Geometry check sheet. Reference: the model listing, model coordinates, mm. A direction names the side the tool comes from. Coordinates: 2 decimals unless noted, no trailing zeros. Write each loop counter-clockwise with the first axis right and the second up, starting at its lowest first coordinate (ties: lowest second). Pieces come first, ordered by that corner, then holes.
from build123d import *

# Parameters (mm, degrees)
BOSS_EXTRUDE1_DEPTH             = 15
SKETCH4_R                       = 10.5
CUT_EXTRUDE2_DEPTH              = 2
M3_CLEARANCE_HOLE2_D            = 3.4
M3X0_5_TAPPED_HOLE1_D           = 2.5
M3X0_5_TAPPED_HOLE1_CSINK_D     = 10
M3X0_5_TAPPED_HOLE1_CSINK_ANGLE = 90


with BuildPart() as part:
    # Sketch1 → Boss-Extrude1 (new body)
    with BuildSketch(Plane.XY):
        with BuildLine():
            Line((0.6875, 12.48107943), (100.385, 6.989404481))
            ThreePointArc((100.385, 6.989404481), (107, 0), (100.385, -6.989404481))
            Line((100.385, -6.989404481), (0.6875, -12.48107943))
            ThreePointArc((0.6875, -12.48107943), (-12.5, 0), (0.6875, 12.48107943))
        make_face()
    extrude(amount=BOSS_EXTRUDE1_DEPTH)

    # Sketch4 → Cut-Extrude2 (cut)
    with BuildSketch(Plane.XY.offset(15)):
        Circle(SKETCH4_R)
    extrude(amount=-CUT_EXTRUDE2_DEPTH, mode=Mode.SUBTRACT)

    # M3 Clearance Hole2 (through all)
    with Locations(Plane.XY.offset(15)):
        with Locations((100, 0)):
            Hole(M3_CLEARANCE_HOLE2_D / 2)

    # M3x0.5 Tapped Hole1 (through all)
    with Locations(Plane(origin=(0, 0, 0), x_dir=(-1, 0, 0), z_dir=(0, 0, -1))):
        with Locations((0, 0)):
            CounterSinkHole(M3X0_5_TAPPED_HOLE1_D / 2, M3X0_5_TAPPED_HOLE1_CSINK_D / 2, counter_sink_angle=M3X0_5_TAPPED_HOLE1_CSINK_ANGLE)


solid = part.part
1. Sectioned sample at A-A, the plane y = 0. Record the boundary of the cut face in (x, z).
Computed values:
outline: (-12.5, 0) - (-5, 0) - (-1.25, 3.75) - (-1.25, 13) - (-10.5, 13) - (-10.5, 15) - (-12.5, 15) - close; (1.25, 3.75) - (5, 0) - (98.3, 0) - (98.3, 15) - (10.5, 15) - (10.5, 13) - (1.25, 13) - close; (101.7, 0) - (107, 0) - (107, 15) - (101.7, 15) - close
2. Access from +Z, -Z, +X, -X, +Y, -Y to the whole of each face (thin tool, end or side, straight path). Record for faces 1 (the cylindrical face through (10, 3.2, 14)), 2 (the conical face through (-0.31, -1.398, 3.568)).
Computed values:
face 1: +Z
face 2: -Z
3. Sectioned sample at C-C, the plane y = -9.25. Record the boundary of the cut face in (x, z).
Computed values:
outline: (-8.41, 0) - (59.35, 0) - (59.35, 15) - (4.97, 15) - (4.97, 13) - (-4.97, 13) - (-4.97, 15) - (-8.41, 15) - close
4. Sectioned sample at D-D, the plane x = 22. Record the boundary of the cut face in (y, z).
Computed values:
outline: (-11.31, 0) - (11.31, 0) - (11.31, 15) - (-11.31, 15) - close
5. Sectioned sample at B-B, the plane z = 7. Give the number of separate pieces and of enclosed holes in the cut face, and give its area (3 significant figures).
Computed values:
separate pieces: 1
enclosed holes: 2
area: 2,260 mm2
6. Gauge pin test, flat ends, axial feed: pin 1 Ø3 at (x, y) = (0, 0) entering from -Z; pin 2 Ø8 at (x, z) = (40.5, 4.5) entering from -Y; pin 3 Ø2 at (x, y) = (2.5, -3.5) entering from +Z; pin 4 Ø5 at (x, z) = (2, 3.5) entering from -Y. Record the tip position at first contact, or that the pin passes through.
Computed values:
pin 1: stops at z = 3.5
pin 2: stops at y = -10.51
pin 3: stops at z = 13
pin 4: stops at y = -12.5
7. Draft check along Y on faces 3 (the flat face through (48, 0, 15)), 4 (the flat face through (2, 0, 13)), 5 (the cylindrical face through (-0.27, -1.22, 8.44)), 6 (the flat face through (51.2, -9.7, 7.4)). Enter one of: released by +Y, released by -Y, zero draft, split by the parting line, or undercut.
Computed values:
face 3: zero draft
face 4: undercut
face 5: undercut
face 6: released by -Y
8. Thickness scan on line 1 along Z through (x, y) = (-7, -4); line 2 along Y through (x, z) = (100, 10); line 3 along Y through (x, z) = (0, 13.55). Record the ranges inside material, lowest first.
Computed values:
line 1: z = 0 to 13
line 2: y = -7.01 to -1.7, 1.7 to 7.01
line 3: y = -12.5 to -10.5, 10.5 to 12.5
